Autodesk Inventor part; units mm, degrees
ref_plane "YZ Plane" through (0, 0, 0) normal (1, 0, 0) x (0, 1, 0)
ref_plane "XZ Plane" through (0, 0, 0) normal (0, 1, 0) x (-1, 0, 0)
ref_plane "XY Plane" through (0, 0, 0) normal (0, 0, 1) x (1, 0, 0)
sketch "Sketch1" plane through (0, 0, 0) normal (0, 0, 1) x (1, 0, 0)
  line L0 (-10.4788, 3.5567) -> (22.1748, -35.3584)
  line L1 (-10.4788, 3.5567) -> (40.3212, 3.5567) construction
  line L2 (22.1748, -35.3584) -> (8.205, -87.4942)
  line L3 (8.205, -87.4942) -> (134.8162, -28.4545)
  line L4 (134.8162, -28.4545) -> (93.9992, 20.1894)
  line L5 (93.9992, 20.1894) -> (-10.4788, 3.5567)
  point P0 (0, 0)
  dimension "d0" = 50.8
  dimension "d1" = 50
  dimension "d2" = 53.975
  dimension "d3" = 125
  dimension "d4" = 139.7
  dimension "d5" = 50
  dimension "d6" = 63.5
  dimension "d7" = 75
extrude "Extrusion1" add sketch "Sketch1" along normal blind 3.175
sketch "Sketch2" plane through (0, 0, 3.175) normal (0, 0, 1) x (1, 0, 0)
  line L0 (-10.4788, 3.5567) -> (22.1748, -35.3584)
  line L1 (22.1748, -35.3584) -> (8.205, -87.4942)
  line L2 (22.1748, -35.3584) -> (9.9297, -20.7652)
  line L3 (22.1748, -35.3584) -> (17.2443, -53.7593)
  line L4 (9.9297, -20.7652) -> (3.7302, -22.1396)
  line L5 (17.2443, -53.7593) -> (11.0448, -55.1337)
  line L6 (15.9753, -36.7328) -> (3.7302, -22.1396)
  line L7 (15.9753, -36.7328) -> (11.0448, -55.1337)
  point P0 (0, 0)
  dimension "d10" = 19.05
  dimension "d11" = 19.05
  dimension "d12" = 6.35
  dimension "d13" = 6.35
  dimension "d14" = 6.35
extrude "Extrusion2" add sketch "Sketch2" against normal blind 3.175
sketch "Sketch3" plane through (0, 0, 0) normal (0, 0, -1) x (-1, 0, 0)
  line L0 (-17.2443, -53.7593) -> (-11.0448, -55.1337)
  line L1 (-11.0448, -55.1337) -> (-15.9753, -36.7328)
  line L2 (-15.9753, -36.7328) -> (-3.7302, -22.1396)
  line L3 (-3.7302, -22.1396) -> (-9.9297, -20.7652)
  line L4 (-3.7302, -22.1396) -> (-6.83, -21.4524)
  line L5 (-11.0448, -55.1337) -> (-14.1446, -54.4465)
  line L6 (-14.1446, -54.4465) -> (-19.0751, -36.0456)
  line L7 (-6.83, -21.4524) -> (-19.0751, -36.0456)
  point P0 (0, 0)
  dimension "d17" = 3.175
  dimension "d18" = 3.175
extrude "Extrusion3" add sketch "Sketch3" along normal blind 12.7
sketch "Sketch4" plane through (3.7302, -22.1396, -12.7) normal (-0.7660444, -0.6427876, 0) x (0, 0, 1)
  line L0 (0, -19.05) -> (0, 0)
  line L1 (15.875, -19.05) -> (0, -19.05)
  line L2 (0, -9.525) -> (6.35, -9.525)
  point P0 (12.7, 19.3577)
  dimension "d21" = 6.35
hole "Hole1" at (9.8528, -29.4362, -6.35) direction (0.7660444, 0.6427876, 0) diameter 6.35 end through all
sketch "Sketch5" plane through (15.9753, -36.7328, -12.7) normal (-0.9659258, 0.258819, 0) x (0, 0, 1)
  line L0 (0, -19.05) -> (0, 0)
  line L1 (15.875, -19.05) -> (0, -19.05)
  line L2 (0, -9.525) -> (6.35, -9.525)
  point P0 (12.7, 31.3464)
  dimension "d29" = 6.35
hole "Hole2" at (13.5101, -45.9332, -6.35) direction (0.9659258, -0.258819, 0) diameter 6.35 end through all
sketch "Sketch6" plane through (0, 0, 0) normal (0, 0, -1) x (-1, 0, 0)
  line L0 (-134.8162, -28.4545) -> (-93.9992, 20.1894)
  line L1 (-114.4077, -4.1326) -> (-103.5422, 8.8164)
  line L2 (-114.4077, -4.1326) -> (-125.2732, -17.0815)
  line L3 (-125.2732, -17.0815) -> (-130.1376, -12.9998)
  line L4 (-130.1376, -12.9998) -> (-108.4066, 12.8981)
  line L5 (-108.4066, 12.8981) -> (-103.5422, 8.8164)
  point P0 (0, 0)
  dimension "d37" = 16.9037
  dimension "d38" = 16.9037
  dimension "d39" = 6.35
  dimension "d40" = 33.8074
extrude "Extrusion4" add sketch "Sketch6" against normal blind 3.175
sketch "Sketch7" plane through (0, 0, 0) normal (0, 0, -1) x (-1, 0, 0)
  line L0 (-103.5422, 8.8164) -> (-108.4066, 12.8981)
  line L1 (-108.4066, 12.8981) -> (-130.1376, -12.9998)
  line L2 (-130.1376, -12.9998) -> (-125.2732, -17.0815)
  line L3 (-108.4066, 12.8981) -> (-130.1376, -12.9998)
  line L4 (-130.1376, -12.9998) -> (-127.7054, -15.0407)
  line L5 (-127.7054, -15.0407) -> (-105.9744, 10.8573)
  line L6 (-105.9744, 10.8573) -> (-108.4066, 12.8981)
  point P0 (0, 0)
  dimension "d43" = 3.175
extrude "Extrusion5" add sketch "Sketch7" along normal blind 12.7
sketch "Sketch8" plane through (108.4066, 12.8981, 3.175) normal (0.7660444, 0.6427876, 0) x (0, 0, -1)
  line L0 (15.875, 0) -> (15.875, -33.8074)
  line L1 (15.875, -16.9037) -> (9.525, -16.9037)
  point P0 (3.175, 59.8019)
  dimension "d46" = 6.35
hole "Hole3" at (119.2721, -0.0509, -6.35) direction (-0.7660444, -0.6427876, 0) diameter 6.35 end through all
sketch "Sketch9" plane through (0, 0, 3.175) normal (0, 0, 1) x (1, 0, 0)
  line L0 (130.1376, -12.9998) -> (108.4066, 12.8981)
  line L1 (103.5422, 8.8164) -> (93.9992, 20.1894)
  line L2 (93.9992, 20.1894) -> (-10.4788, 3.5567)
  line L3 (71.6563, 16.6324) -> (76.7318, -15.2495)
  line L4 (111.0345, 9.7664) -> (80.0581, -16.2259)
  line L5 (80.0581, -16.2259) -> (74.7441, -9.893)
  line L6 (76.7318, -15.2495) -> (78.9434, -14.8974)
  line L7 (17.2443, -53.7593) -> (8.205, -87.4942)
  line L8 (11.0448, -55.1337) -> (34.2557, 31.4904)
  line L9 (78.9434, -14.8974) -> (25.6522, -0.6181)
  line L10 (78.9434, -14.8974) -> (82.2304, -2.6302)
  point P0 (0, 0)
  dimension "d54" = 32.2834
  dimension "d55" = 40.4368
  dimension "d71" = 12.7
hole "Hole6" at (82.2304, -2.6302, 3.175) direction (0, 0, -1) diameter 7.9375 end through all
properties part number "Right Bicep"
Verification items for the finished model (mm, model axes). A direction names the side the tool comes from. Coordinates: 2 decimals unless noted, no trailing zeros. Order: outer loops, then holes, each group sorted by start corner. A loop starts at its lowest first (then second) coordinate and runs counter-clockwise, first axis right, second up. Notation, with made-up numbers: (47, 54.25) - (84, 54.25) arc R20 cw to (84, 92.25) - close; hole circle Ø3 at (25, 4.5). An arc over 180 degrees is marked (long way). Return JSON: item names as keys, results as strings.
(1) Section check A-A, the plane z = -6. Record the cut outline in (x, y).
Filled sheet:
{"outline": "(3.73, -22.14) - (7.82, -27.02) - (9.98, -25.21) - (6.83, -21.45) - close; (11.04, -55.13) - (14.14, -54.45) - (15.41, -49.71) - (12.69, -48.98) - close; (11.88, -31.85) - (15.98, -36.73) - (14.33, -42.89) - (17.05, -43.61) - (19.08, -36.05) - (14.04, -30.04) - close; (105.97, 10.86) - (114.81, 0.33) - (117.24, 2.37) - (108.41, 12.9) - close; (118.87, -4.51) - (127.71, -15.04) - (130.14, -13) - (121.3, -2.47) - close"}
(2) Thickness scan on line 1 along Z through (x, y) = (9, -19) (3 decimals); line 2 along Y through (x, z) = (4.5, -3); line 3 along Y through (x, z) = (118, -1.5). Record the ranges inside material, lowest first.
Filled sheet:
{"line 1": "z = 0 to 3.175", "line 2": "y = -23.06 to -21.97", "line 3": "y = -3.47 to 1.47"}
(3) Section check C-C, the plane y = -64.5. Record the cut outline in (x, z) (3 decimals).
Filled sheet:
{"outline": "(14.366, 0) - (57.516, 0) - (57.516, 3.175) - (14.366, 3.175) - close"}
(4) Go/stop test with flat-tipped pins: pin 1 (1 mm diameter, centred on x = 43.5, z = 1, fed in from -Y); pin 2 (5 mm diameter, centred on y = -67.5, z = 0.5, fed in from -X); pin 3 (5 mm diameter, centred on y = -24, z = -9, fed in from +X); pin 4 (6.5 mm diameter, centred on x = 82.23, y = -2.63, fed in from +Z). Record where each tip stops, or that it passes through.
Filled sheet:
{"pin 1": "stops at y = -71.27", "pin 2": "stops at x = 12.89", "pin 3": "stops at x = 11.06", "pin 4": "passes through"}
(5) Section check D-D, the plane x = 111.5. Record the cut outline in (y, z) (3 decimals), and give its area (3 significant figures).
Filled sheet:
{"outline": "(-39.327, 0) - (4.272, 0) - (4.272, -12.7) - (9.212, -12.7) - (9.212, 3.175) - (-39.327, 3.175) - close", "area": "217 mm^2"}
(6) Mould release check, pull along X, two halves, no side actions. Record for faces 4 (the flat face through (61, -21, 0)), 5 (the flat face through (119.12, 0.13, -2.89)), 6 (the flat face through (98.84, 14.42, 1.57)), 7 (the flat face through (13.476, -46.062, -2.887)): pulls with the +X half, pulls with the -X half, needs draft (parallel to the pull), parting line crosses it, or undercut.
Filled sheet:
{"face 4": "needs draft", "face 5": "pulls with the +X half", "face 6": "undercut", "face 7": "pulls with the -X half"}
(7) Section check B-B, the plane x = 65.5. Record the cut outline in (y, z) (3 decimals), and give its area (3 significant figures).
Filled sheet:
{"outline": "(-60.777, 0) - (15.652, 0) - (15.652, 3.175) - (-60.777, 3.175) - close", "area": "243 mm^2"}
(8) Access from +Z, -Z, +X, -X, +Y, -Y to the whole of each face (thin tool, end or side, straight path). Record for faces 1 (the flat face through (128.28, -14.56, -2.89)), 2 (the flat face through (9.94, -29.54, -2.89)), 3 (the flat face through (114.58, 0.6, -6.26)).
Filled sheet:
{"face 1": "+Z, -Z, +X", "face 2": "+Z, -Z, -X", "face 3": "-Z, -X, -Y"}
